Check sheet for the modelled part. Datum: model origin and axes. Units: mm. A direction names the side the tool comes from. Give positions to 0.01 mm unless a question says otherwise; leave off trailing zeros. Loops run counter-clockwise (first coordinate to the right, second up) from the corner with the lowest first, then second, coordinate; pieces in that order, holes last. Notation, with made-up numbers: M 85,14.5 L 142,14.5 A21 ccw 142,53.5 Z; hole C 58.5,83.25 d7. An arc over 180 degrees is marked long. Put each result on its own line as item: value. Start each with the question number.
```python
from build123d import *

# Parameters (mm, degrees)
SKETCH1_R           = 42.3291
SKETCH1_R_2         = 6.35
BOSS_EXTRUDE1_DEPTH = 12.7


with BuildPart() as part:
    # Sketch1 → Boss-Extrude1 (new body)
    with BuildSketch(Plane(origin=(0, 0, 0), x_dir=(1, 0, 0), z_dir=(0, 1, 0))):
        Circle(SKETCH1_R)
        Circle(SKETCH1_R_2, mode=Mode.SUBTRACT)
    extrude(amount=BOSS_EXTRUDE1_DEPTH)

    # Cut-Sweep5: sweep along a path in Sketch3
    with BuildLine(Plane(origin=(0, 12.7, 0), x_dir=(1, 0, 0), z_dir=(0, 1, 0))) as cut_sweep5_path:
        CenterArc((0, 0), 25.4, 0, 360)
    # Sketch4 → Cut-Sweep5 (sweep, cut)
    with BuildSketch(Plane.XY):
        with BuildLine():
            Line((-31.75, 12.7), (-19.05, 12.7))
            Line((-19.05, 12.7), (-19.05, 10.16))
            ThreePointArc((-19.05, 10.16), (-19.793948776, 8.363948776), (-21.59, 7.62))
            Line((-21.59, 7.62), (-29.21, 7.62))
            ThreePointArc((-29.21, 7.62), (-31.006051224, 8.363948776), (-31.75, 10.16))
            Line((-31.75, 10.16), (-31.75, 12.7))
        make_face()
    sweep(path=cut_sweep5_path.line, mode=Mode.SUBTRACT)


solid = part.part
```
Q1. Thickness scan on line 1 along Z through (x, y) = (0, 11.6); line 2 along X through (y, z) = (8.75, -10.5); line 3 along X through (y, z) = (8.25, 0). Record the ranges inside material, lowest first. Write a range as [from, to].
Q2. Depth check by flat-ended pin: P1, Ø11.5, axis at x = 0, z = 0, coming from the +Y side; P2, Ø4, axis at x = 28, y = 7.5, coming from the -Z side; P3, Ø5, axis at y = 8, z = 7.5, coming from the +X side; P4, Ø3, axis at x = -22.5, y = 2.5, coming from the -Z side. Enter the tip coordinate at first touch or a pass-through.
Q3. Mould release check, pull along X, two halves, no side actions. Record for faces 1 (the face through (-1, 0, 9)), 2 (the face through (-4.13, 11.448, 18.597)), 3 (the face through (40.374, 6.261, -12.715)): pulls with the +X half, pulls with the -X half, needs draft (parallel to the pull), parting line crosses it, or undercut.
Q4. Section check A-A, the plane y = 2.75. Record the cut outline in (x, z).
Q5. Section check B-B, the plane z = 36.5. Record the cut outline in (x, y), then the cut area to 3 significant figures.
Q6. Access from +Z, -Z, +X, -X, +Y, -Y to the whole of each face (thin tool, end or side, straight path). Record for faces 4 (the face through (-6.883, 11.412, 30.995)), 5 (the face through (-1.38, 6.26, 6.2)).
Found:
1. line 1: z = [-42.33, -31.75], [-19.05, -6.35], [6.35, 19.05], [31.75, 42.33]
1. line 2: x = [-41.01, -29.51], [-16.4, 16.4], [29.51, 41.01]
1. line 3: x = [-42.33, -30.88], [-19.92, -6.35], [6.35, 19.92], [30.88, 42.33]
2. P1: passes through
2. P2: stops at z = -33.4
2. P3: stops at x = 42.03
2. P4: stops at z = -36.75
3. face 1: needs draft
3. face 2: undercut
3. face 3: parting line crosses it
4. outline: C 0,0 d84.66; hole C 0,0 d12.7
5. outline: M -21.44,0 L 21.44,0 L 21.44,12.7 L -21.44,12.7 Z
5. area: 544 mm^2
6. face 4: +Y
6. face 5: +Y, -Y
